For this review, take the finished solid that the model builds, in its own axes (mm). A direction names the side the tool comes from. Round coordinates to 2 decimals unless told otherwise and drop trailing zeros. Order: outer loops, then holes, each group sorted by start corner. A loop starts at its lowest first (then second) coordinate and runs counter-clockwise, first axis right, second up.
```python
from build123d import *

# Parameters (mm, degrees)
BOSS_EXTRUDE1_DEPTH = 5
BOSS_EXTRUDE2_DEPTH = 33


with BuildPart() as part:
    # Sketch1 → Boss-Extrude1 (new body)
    with BuildSketch(Plane(origin=(0, 0, 0), x_dir=(1, 0, 0), z_dir=(0, 1, 0))):
        with BuildLine():
            Line((-10.5, 48.885069295), (-8.5, 77.211291854))
            ThreePointArc((-8.5, 77.211291854), (-7.552703541, 79.194752328), (-5.507449958, 80))
            Line((-5.507449958, 80), (5.507449958, 80))
            ThreePointArc((5.507449958, 80), (7.552703541, 79.194752328), (8.5, 77.211291854))
            Line((8.5, 77.211291854), (10.5, 48.885069295))
            ThreePointArc((10.5, 48.885069295), (50, 0), (10.5, -48.885069295))
            Line((10.5, -48.885069295), (8.5, -77.211291854))
            ThreePointArc((8.5, -77.211291854), (7.552703541, -79.194752328), (5.507449958, -80))
            Line((5.507449958, -80), (-5.507449958, -80))
            ThreePointArc((-5.507449958, -80), (-7.552703541, -79.194752328), (-8.5, -77.211291854))
            Line((-8.5, -77.211291854), (-10.5, -48.885069295))
            ThreePointArc((-10.5, -48.885069295), (-50, 0), (-10.5, 48.885069295))
        make_face()
    extrude(amount=BOSS_EXTRUDE1_DEPTH)

    # Sketch2 → Boss-Extrude2 (add)
    with BuildSketch(Plane(origin=(0, 0, 0), x_dir=(1, 0, 0), z_dir=(0, 1, 0))):
        with BuildLine():
            Line((-154, -40), (-69.5, -40))
            ThreePointArc((-69.5, -40), (-62, -47.5), (-54.5, -40))
            Line((-54.5, -40), (-31, -40))
            ThreePointArc((-31, -40), (-26.757359313, -38.242640687), (-25, -34))
            Line((-25, -34), (-25, 34))
            ThreePointArc((-25, 34), (-26.757359313, 38.242640687), (-31, 40))
            Line((-31, 40), (-54.5, 40))
            ThreePointArc((-54.5, 40), (-62, 47.5), (-69.5, 40))
            Line((-69.5, 40), (-154, 40))
            ThreePointArc((-154, 40), (-164.606601718, 35.606601718), (-169, 25))
            Line((-169, 25), (-169, -25))
            ThreePointArc((-169, -25), (-164.606601718, -35.606601718), (-154, -40))
        make_face()
    extrude(amount=BOSS_EXTRUDE2_DEPTH)


solid = part.part
```
Q1. Clearance check with flat-ended pins moving along their axes: pin 1 (14 mm diameter, centred on y = 19.5, z = -15.5, fed in from +X); pin 2 (8 mm diameter, centred on y = 16.5, z = -41.5, fed in from +X); pin 3 (19 mm diameter, centred on x = -48.5, y = 13.5, fed in from +Z); pin 4 (12 mm diameter, centred on x = 6.5, z = -44, fed in from -Y). State where each tip first meets the part, or that it passes through.
Q2. Tool access review of faces 4 (the face through (-20.646, 2.465, 45.539)), 5 (the face through (9.514, 2.465, 62.85)), 6 (the face through (-25, 19, 0)): name each direction out of +Z, -Z, +X, -X, +Y, -Y from which nothing blocks a thin tool from reaching the whole face with its end or side.
Q3. Take a section at B-B, the plane y = 30. State the section outline as (x, z) points.
Q4. Take a section at D-D, the plane x = -62. State the section outline as (y, z) points, plus the area to 4 significant figures.
Q5. Mouldability with a two-part tool opening along X and no side actions: class faces 1 (the face through (-164.49, 16.27, -35.72)), 2 (the face through (-20.922, 2.465, -45.412)), 3 (the face through (-112, 16, 40)) as +X half, -X half, draft (parallel to the pull), parting line (faces both ways), or undercut.
Q6. Take a section at C-C, the plane z = 44. State the section outline as (x, y) points.
Q7. Wall thickness on line 1 (Z direction, x = -126.5, y = 14.5); line 2 (X direction, y = 10, z = 13.5); line 3 (X direction, y = 3.5, z = 49): over which ranges is each line inside the solid? List them lowest first.
Q8. Take a section at A-A, the plane z = 1. State the section outline as (x, y) points, plus the area to 3 significant figures.
Working result:
1. pin 1: stops at x = -25
1. pin 2: stops at x = -26.13
1. pin 3: stops at z = 46.34
1. pin 4: stops at y = 0
2. face 4: +Z, +Y, -Y
2. face 5: +Z, +X, +Y, -Y
2. face 6: +Z, -Z, +X, +Y
3. outline: (-169, -25) arc R15 ccw to (-154, -40) - (-69.5, -40) arc R7.5 ccw to (-54.5, -40) - (-31, -40) arc R6 ccw to (-25, -34) - (-25, 34) arc R6 ccw to (-31, 40) - (-54.5, 40) arc R7.5 ccw to (-69.5, 40) - (-154, 40) arc R15 ccw to (-169, 25) - close
4. outline: (0, -47.5) - (33, -47.5) - (33, 47.5) - (0, 47.5) - close
4. area: 3,135 mm2
5. face 1: -X half
5. face 2: undercut
5. face 3: draft
6. outline: (-68.34, 0) - (-55.66, 0) - (-55.66, 33) - (-68.34, 33) - close; (-23.75, 0) - (23.75, 0) - (23.75, 5) - (-23.75, 5) - close
7. line 1: z = -40 to 40
7. line 2: x = -169 to -25
7. line 3: x = -10.49 to 10.49
8. outline: (-169, 0) - (49.99, 0) - (49.99, 5) - (-25, 5) - (-25, 33) - (-169, 33) - close
8. area: 5,130 mm2
